from build123d import *

# Parameters (mm, degrees)
F1_DEPTH = 25.4


with BuildPart() as f1:
    # F0 (on Front) → F1 (new body)
    with BuildSketch(Plane.XZ):
        with BuildLine():
            Line((-36.472339, 67.40699), (-66.070311, 67.597948))
            Line((-66.070311, 67.597948), (-66.070311, 16.80401))
            Line((-66.070311, 16.80401), (-15.276372, 16.80401))
            Line((-15.276372, 16.80401), (-15.276372, 42.200983))
            ThreePointArc((-15.276372, 42.200983), (-30.809465, 50.654006), (-36.472339, 67.40699))
        make_face()
    extrude(amount=F1_DEPTH)


solid = f1.part
Geometry: final body of the model. Coordinates: model frame, mm. Round coordinates to 2 decimals unless told otherwise and drop trailing zeros. Loops run counter-clockwise (first coordinate to the right, second up) from the corner with the lowest first, then second, coordinate; pieces in that order, holes last. Notation, with made-up numbers: (14, -10) - (47, -10) arc R19 ccw to (47, 24) - close; hole circle Ø4 at (65, 21). An arc over 180 degrees is marked (long way). Write each question's results on one line, items separated by ' | '. Start each with the question number.
1) Cut plane B-B on z = 49.5. Return loops of the section in (x, y), then the cut area to 3 significant figures.
2) Cut plane C-C on x = -25.5. Return loops of the section in (y, z).
3) Cut plane A-A on y = -7.75. Return loops of the section in (x, z).
4) First-contact query: P1, Ø1.5, axis at x = -38, y = -13.5, coming from the +Z side; P2, Ø1, axis at y = -4, z = 62.5, coming from the +X side; P3, Ø3, axis at x = -32, y = -21, coming from the +Z side. Flat tips, straight axial feed; report the tip coordinate or a pass-through.
5) Line query: probe 1 along Z at (x, y) = (-38.5, -4); probe 2 along X at (y, z) = (-4.5, 56); probe 3 along Z at (x, y) = (-18.5, -11.25). Output: solid intervals per line, ascending. Write a range as [from, to].
6) Mould query, pull axis Y, two halves, no side actions, for faces 1 (the face through (-47, -25.4, 37)), 2 (the face through (-47, 0, 37)), 3 (the face through (-41, -13, 16.804)). Classes: released by +Y, released by -Y, zero draft, split by the parting line, or undercut.
Verdict:
1) outline: (-66.07, -25.4) - (-29.77, -25.4) - (-29.77, 0) - (-66.07, 0) - close | area: 922 mm2
2) outline: (-25.4, 16.8) - (0, 16.8) - (0, 45.95) - (-25.4, 45.95) - close
3) outline: (-66.07, 16.8) - (-15.28, 16.8) - (-15.28, 42.2) arc R24.25 cw to (-36.47, 67.41) - (-66.07, 67.6) - close
4) P1: stops at z = 67.42 | P2: stops at x = -36.12 | P3: stops at z = 54.58
5) probe 1: z = [16.8, 67.42] | probe 2: x = [-66.07, -34.22] | probe 3: z = [16.8, 42.83]
6) face 1: released by -Y | face 2: released by +Y | face 3: zero draft
